Part model, mm, in its own coordinate system. A direction names the side the tool comes from. Give positions to 0.01 mm unless a question says otherwise; leave off trailing zeros. Write each loop counter-clockwise with the first axis right and the second up, starting at its lowest first coordinate (ties: lowest second). Pieces come first, ordered by that corner, then holes.
from build123d import *

# Parameters (mm, degrees)
TROU_TARAUD_M42_D     = 3.3
TROU_TARAUD_M42_DEPTH = 11.1
TROU_TARAUD_M42_TIP   = 0.991420021


with BuildPart() as part:
    # Esquisse1 → Révolution1 (revolve)
    with BuildSketch(Plane.XY, mode=Mode.PRIVATE) as r_volution1_sk:
        Polygon((0, 0), (0, 4), (13, 4), (13, 5.5), (25, 5.5), (25, 9), (29, 9), (29, 5.5), (50, 5.5), (50, 3.5), (53, 3.5), (55.5, 6), (111.5, 6), (112.5, 5), (112.5, 0), align=None)
    revolve(r_volution1_sk.sketch.rotate(Axis((-83.694243421, 0, 0), (1, 0, 0)), 90), axis=Axis((-83.694243421, 0, 0), (1, 0, 0)))

    # Trou taraudé M42
    with Locations(Plane.ZY):
        with Locations((0, 0)):
            Hole(TROU_TARAUD_M42_D / 2, depth=TROU_TARAUD_M42_DEPTH)
            with Locations((0, 0, -(TROU_TARAUD_M42_DEPTH + TROU_TARAUD_M42_TIP / 2))):  # 118° drill point
                Cone(0, TROU_TARAUD_M42_D / 2, TROU_TARAUD_M42_TIP, mode=Mode.SUBTRACT)


solid = part.part
1) Mould opens along X. For faces 4 (the conical face through (53.156, 3.244, 1.687)), 5 (the flat face through (112.5, 0, 0)), 6 (the cylindrical face through (19.08, 5.37, -1.19)) say: +X half, -X half, draft (parallel to the pull), parting line (faces both ways), or undercut.
Check result:
face 4: undercut
face 5: +X half
face 6: draft
2) 3-axis set-ups, long thin cutter, end or side, ignore diameter. For faces 1 (the cylindrical face through (83.892, -1.802, 5.723)), 2 (the cylindrical face through (39.65, 5.37, -1.19)), 3 (the flat face through (13, 2, 4)): which of +Z, -Z, +X, -X, +Y, -Y reach the whole face in a straight line?
Check result:
face 1: +X
face 2: none
face 3: -X
3) Saw through at A-A (x = 92). Write the cut outline in (y, z), and give its area (3 significant figures).
Check result:
outline: circle Ø12 at (0, 0)
area: 113 mm2
4) Saw through at B-B (x = 16.5). Write the cut outline in (y, z).
Check result:
outline: circle Ø11 at (0, 0)
5) Drill centre lines: L1, parallel to Y at x = 4.5, z = 0; L2, parallel to X at y = 2.5, z = 8.5; L3, parallel to X at y = 2, z = -5.5. Where is each one in solid material? Low to high.
Check result:
L1: y = -4 to -1.65, 1.65 to 4
L2: x = 25 to 29
L3: x = 25 to 29, 55.35 to 111.65
6) Flat gauge pins, fed straight in: P1, Ø2.5, axis at y = 0, z = 0, coming from the -X side; P2, Ø4, axis at x = 54, z = 4.5, coming from the +Y side; P3, Ø8, axis at x = 14.5, z = -7, coming from the +Y side. Where does each tip first touch, or does it go through?
Check result:
P1: stops at x = 11.34
P2: stops at y = 5.09
P3: stops at y = 4.61
